The model under review builds one solid part; all positions refer to its coordinate system, in mm. Face numbers are marked on the shaded views. A direction names the side the tool comes from. Round coordinates to 2 decimals unless told otherwise and drop trailing zeros. Order: outer loops, then holes, each group sorted by start corner. A loop starts at its lowest first (then second) coordinate and runs counter-clockwise, first axis right, second up. Notation, with made-up numbers: (-15.5, 40.25) -> (21.5, 40.25) arc R10 cw to (21.5, 47.25) -> close; hole circle Ø5 at (84, 49). An arc over 180 degrees is marked (long way). Use a Markdown table: item, result. Add a question column.
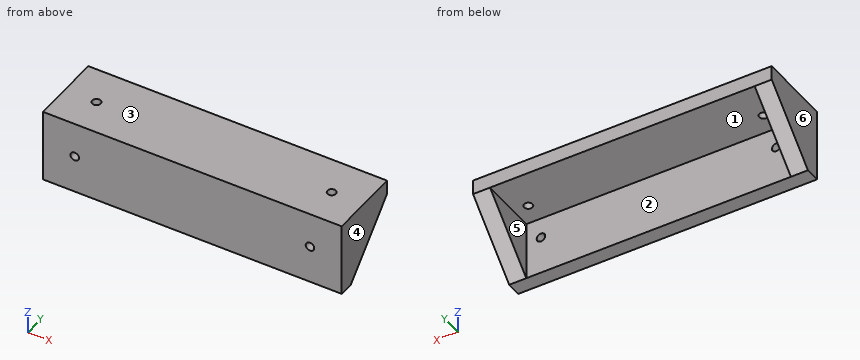
```python
from build123d import *

# Parameters (mm, degrees)
BOSS_EXTRUDE1_START = -50.8
BOSS_EXTRUDE1_DEPTH = 101.6
HOLLOW_START        = 45
SKETCH3_W           = 20
SKETCH3_H           = 20
HOLLOW_DEPTH        = 90
BOTTOM_HOLES_D      = 2.9
FRONT_HOLES_D       = 2.9


with BuildPart() as part:
    # Sketch1 → Boss-Extrude1 (new body)
    with BuildSketch(Plane(origin=(0, 0, 0), x_dir=(0, 0, -1), z_dir=(1, 0, 0)).offset(BOSS_EXTRUDE1_START)):
        Polygon((0, 25), (0, 0), (25, 0), (25, 5), (5, 25), align=None)
    extrude(amount=BOSS_EXTRUDE1_DEPTH)

    # Sketch3 → hollow (cut)
    with BuildSketch(Plane(origin=(0, 0, 0), x_dir=(0, 0, -1), z_dir=(1, 0, 0)).offset(HOLLOW_START)):
        with Locations((15, 15)):
            Rectangle(SKETCH3_W, SKETCH3_H)
    extrude(amount=-HOLLOW_DEPTH, mode=Mode.SUBTRACT)

    # bottom holes (through all)
    with Locations(Plane(origin=(0, 0, 0), x_dir=(-1, 0, 0), z_dir=(0, -1, 0))):
        with Locations((40, 12), (-40, 12)):
            Hole(BOTTOM_HOLES_D / 2)

    # front holes (through all)
    with Locations(Plane.XY):
        with Locations((-40, 12), (40, 12)):
            Hole(FRONT_HOLES_D / 2)


solid = part.part
```
Q1. For pin 1 (8 mm diameter, centred on x = -19.5, y = 14, fed in from -Z); pin 2 (2.5 mm diameter, centred on x = 40, y = 12, fed in from +Z); pin 3 (10 mm diameter, centred on x = 9, z = -21.5, fed in from +Y), all flat-tipped, find the tip position at first contact; note any pin that passes through.
Q2. Add section C-C, the plane z = -12. Give the boundary of the cut face in (x, y).
Q3. For the marked faces 5 and 6, list the 3-axis set-ups (+Z, -Z, +X, -X, +Y, -Y) from which the entire face can be reached by the end or side of a thin tool; tool diameter is ignored.
Q4. Draft analysis for pull direction X (two halves, no side actions). For the marked faces 1, 2, 3 and 4, state which applies: released by +X, released by -X, zero draft, split by the parting line, or undercut.
Q5. To check wall thickness, follow line 1 along X through (y, z) = (1.1, -12); line 2 along Y through (x, z) = (40, -2.95); line 3 along Z through (x, y) = (40, 2.55). State the ranges of each line that lie inside material, in increasing order.
Q6. Add section D-D, the plane z = -21.5. Give the boundary of the cut face in (x, y).
Q7. Add section B-B, the plane x = 40. Give the boundary of the cut face in (y, z).
Q8. Add section A-A, the plane y = 12. Give the boundary of the cut face in (x, z).
Return value:
| question | item | result |
|---|---|---|
| 1 | pin 1 | z = -5 |
| 1 | pin 2 | through |
| 1 | pin 3 | y = 5 |
| 2 | outline | (-50.8, 0) -> (-41.45, 0) -> (-41.45, 5) -> (-45, 5) -> (-45, 18) -> (-50.8, 18) -> close; (-38.55, 0) -> (38.55, 0) -> (38.55, 5) -> (-38.55, 5) -> close; (41.45, 0) -> (50.8, 0) -> (50.8, 18) -> (45, 18) -> (45, 5) -> (41.45, 5) -> close |
| 3 | face 5 | -Z, +Y |
| 3 | face 6 | +Z, -Z, -X, +Y, -Y |
| 4 | face 1 | undercut |
| 4 | face 2 | undercut |
| 4 | face 3 | zero draft |
| 4 | face 4 | released by +X |
| 5 | line 1 | -50.8 to -41.45, -38.55 to 38.55, 41.45 to 50.8 |
| 5 | line 2 | 0 to 10.55, 13.45 to 25 |
| 5 | line 3 | -25 to -13.45, -10.55 to 0 |
| 6 | outline | (-50.8, 0) -> (50.8, 0) -> (50.8, 8.5) -> (45, 8.5) -> (45, 5) -> (-45, 5) -> (-45, 8.5) -> (-50.8, 8.5) -> close |
| 7 | outline | (0, -25) -> (5, -25) -> (5, -13.45) -> (0, -13.45) -> close; (0, -10.55) -> (5, -10.55) -> (5, -5) -> (10.55, -5) -> (10.55, 0) -> (0, 0) -> close; (13.45, -5) -> (25, -5) -> (25, 0) -> (13.45, 0) -> close |
| 8 | outline | (-50.8, -18) -> (-45, -18) -> (-45, -5) -> (-41.45, -5) -> (-41.45, 0) -> (-50.8, 0) -> close; (-38.55, -5) -> (38.55, -5) -> (38.55, 0) -> (-38.55, 0) -> close; (41.45, -5) -> (45, -5) -> (45, -18) -> (50.8, -18) -> (50.8, 0) -> (41.45, 0) -> close |
